```python
from build123d import *

# Parameters (mm, degrees)
EXTRUDE_1_DEPTH = 16.5
SKETCH_2_R      = 0.3
EXTRUDE_2_DEPTH = 8
SKETCH_3_R      = 0.3
EXTRUDE_3_DEPTH = 8


with BuildPart() as part:
    # Эскиз1 → Бобышка-Вытянуть1 (new body)
    with BuildSketch(Plane.XY):
        with BuildLine():
            Line((-2.35, -3.85), (2.35, -3.85))
            ThreePointArc((2.35, -3.85), (3.410660172, -3.410660172), (3.85, -2.35))
            Line((3.85, -2.35), (3.85, 2.35))
            ThreePointArc((3.85, 2.35), (3.410660172, 3.410660172), (2.35, 3.85))
            Line((2.35, 3.85), (-2.35, 3.85))
            ThreePointArc((-2.35, 3.85), (-3.410660172, 3.410660172), (-3.85, 2.35))
            Line((-3.85, 2.35), (-3.85, -2.35))
            ThreePointArc((-3.85, -2.35), (-3.410660172, -3.410660172), (-2.35, -3.85))
        make_face()
    extrude(amount=EXTRUDE_1_DEPTH)

    # Эскиз2 → Бобышка-Вытянуть2 (add)
    with BuildSketch(Plane(origin=(0, 0, 0), x_dir=(-1, 0, 0), z_dir=(0, 0, -1))):
        with Locations((-2.5, -2.5)):
            Circle(SKETCH_2_R)
        with Locations((2.5, -2.5)):
            Circle(SKETCH_2_R)
    extrude(amount=EXTRUDE_2_DEPTH)

    # Эскиз3 → Бобышка-Вытянуть3 (add)
    with BuildSketch(Plane.XY.offset(16.5)):
        with Locations((2.5, -2.5)):
            Circle(SKETCH_3_R)
        with Locations((-2.5, 2.5)):
            Circle(SKETCH_3_R)
    extrude(amount=EXTRUDE_3_DEPTH)


solid = part.part
```
Work out the finished part from the listing and answer in its coordinate system (mm). Give positions to 0.01 mm unless a question says otherwise; leave off trailing zeros. Order: outer loops, then holes, each group sorted by start corner. A loop starts at its lowest first (then second) coordinate and runs counter-clockwise, first axis right, second up. Notation, with made-up numbers: (-13.5, -13.75) - (32.5, -13.75) arc R24 ccw to (32.5, 9.25) - close; hole circle Ø6 at (53.25, 73). An arc over 180 degrees is marked (long way). One line per item, written item: value. Start each with the question number.
1. Section C-C, the plane y = 1 is taken. Write down the section's boundary in (x, z).
2. Each of these flat-tipped pins is pushed along its axis until it touches: pin 1 Ø1 at (y, z) = (-2, 18.5) entering from +X; pin 2 Ø4 at (y, z) = (2.5, 19) entering from -X; pin 3 Ø2.5 at (x, y) = (1, 0) entering from -Z. Where does it stop, or does it pass through?
3. Consider line 1 (Z direction, x = 0.75, y = -1.5); line 2 (Y direction, x = 2.5, z = 9); line 3 (X direction, y = -2.75, z = -1.5). Determine where each line is inside the solid, lowest interval first.
4. Section A-A, the plane z = 13 is taken. Write down the section's boundary in (x, y).
5. Section B-B, the plane z = 21.5 is taken. Write down the section's boundary in (x, y), then the cut area to 3 significant figures.
Filled sheet:
1. outline: (-3.85, 0) - (3.85, 0) - (3.85, 16.5) - (-3.85, 16.5) - close
2. pin 1: x = 2.8
2. pin 2: x = -2.8
2. pin 3: z = 0
3. line 1: 0 to 16.5
3. line 2: -3.84 to 3.84
3. line 3: -2.67 to -2.33, 2.33 to 2.67
4. outline: (-3.85, -2.35) arc R1.5 ccw to (-2.35, -3.85) - (2.35, -3.85) arc R1.5 ccw to (3.85, -2.35) - (3.85, 2.35) arc R1.5 ccw to (2.35, 3.85) - (-2.35, 3.85) arc R1.5 ccw to (-3.85, 2.35) - close
5. outline: circle Ø0.6 at (-2.5, 2.5); circle Ø0.6 at (2.5, -2.5)
5. area: 0.565 mm²
